Part model, mm, in its own coordinate system. A direction names the side the tool comes from. Round coordinates to 2 decimals unless told otherwise and drop trailing zeros. Loops run counter-clockwise (first coordinate to the right, second up) from the corner with the lowest first, then second, coordinate; pieces in that order, holes last. Notation, with made-up numbers: (11.25, 40) -> (64.25, 40) arc R30 ccw to (64.25, 78) -> close; hole circle Ø1 at (-9, 13). An arc over 180 degrees is marked (long way). Answer as CSV lines item,"result".
from build123d import *

# Parameters (mm, degrees)
BOSS_EXTRUDE1_DEPTH                      = 12.7
SKETCH5_R                                = 3.4544
CUT_EXTRUDE2_DEPTH                       = 31.760138832
SKETCH6_W                                = 19.05
SKETCH6_H                                = 5.55625
SKETCH7_W                                = 19.05
SKETCH7_H                                = 5.55625
CUT_EXTRUDE3_REACH                       = 49.094
SKETCH8_R                                = 2.2479
CUT_EXTRUDE4_DEPTH                       = 48.544988458
MIRROR1_AT_THE_SECOND_PLANE_COPY_1_DEPTH = 48.544988458


with BuildPart() as part:
    # Sketch2 → Boss-Extrude1 (new, symmetric)
    with BuildSketch(Plane(origin=(0, 0, 0), x_dir=(1, 0, 0), z_dir=(0, 1, 0))):
        Polygon((-19.05, 6.35), (19.05, 6.35), (24.972107259, -6.35), (-24.972107259, -6.35), align=None)
    extrude(amount=BOSS_EXTRUDE1_DEPTH, both=True)

    # Sketch5 → Cut-Extrude2 (cut, through all)
    with BuildSketch(Plane.XY.offset(6.35)):
        Circle(SKETCH5_R)
    extrude(amount=-CUT_EXTRUDE2_DEPTH, mode=Mode.SUBTRACT)

    # Sweep1: sweep along a curve in space
    with BuildLine() as sweep1_path:
        Line((-19.05, 12.7, -6.35), (-24.972107259, 12.7, 6.35))
    # Sketch6 → Sweep1 (sweep)
    with BuildSketch(Plane.XY.offset(6.35)):
        with Locations((-34.497107259, 0)):
            Rectangle(SKETCH6_W, SKETCH6_H)
    sweep(path=sweep1_path.line)

    # Sweep2: sweep along a curve in space
    with BuildLine() as sweep2_path:
        Line((24.972107259, 12.7, 6.35), (19.05, 12.7, -6.35))
    # Sketch7 → Sweep2 (sweep)
    with BuildSketch(Plane.XY.offset(6.35)):
        with Locations((34.497107259, 0)):
            Rectangle(SKETCH7_W, SKETCH7_H)
    sweep(path=sweep2_path.line)

    # Sketch8 → Cut-Extrude3 (cut, up to next)
    with BuildSketch(Plane(origin=(0, 2.778125, 0), x_dir=(1, 0, 0), z_dir=(0, 1, 0)), mode=Mode.PRIVATE) as cut_extrude3_sk1:
        with Locations(Location((-32.520728307, 0, 0), (0, 0, 180))):
            Circle(SKETCH8_R)
    cut_extrude3_tool1 = extrude(cut_extrude3_sk1.sketch, amount=-CUT_EXTRUDE3_REACH, mode=Mode.PRIVATE) & part.part
    # Sketch8 → Cut-Extrude3 (cut, up to next)
    with BuildSketch(Plane(origin=(0, 2.778125, 0), x_dir=(1, 0, 0), z_dir=(0, 1, 0)), mode=Mode.PRIVATE) as cut_extrude3_sk2:
        with Locations(Location((32.520728307, 0, 0), (0, 0, 180))):
            Circle(SKETCH8_R)
    cut_extrude3_tool2 = extrude(cut_extrude3_sk2.sketch, amount=-CUT_EXTRUDE3_REACH, mode=Mode.PRIVATE) & part.part
    add(cut_extrude3_tool1.solids().sort_by_distance((-32.520728, 2.778125, 0))[0], mode=Mode.SUBTRACT)
    add(cut_extrude3_tool2.solids().sort_by_distance((32.520728, 2.778125, 0))[0], mode=Mode.SUBTRACT)

    # Sketch9 → Cut-Extrude4 (cut, through all)
    with BuildSketch(Plane.XY.offset(6.35)):
        with BuildLine():
            Line((-24.972107259, 12.7), (-24.972107259, 7.9375))
            Line((-24.972107259, 7.9375), (-18.622107259, 7.9375))
            Line((-18.622107259, 7.9375), (-3.451726858, 12.221930359))
            ThreePointArc((-3.451726858, 12.221930359), (-1.742338148, 12.579914856), (0, 12.7))
            Line((0, 12.7), (-24.972107259, 12.7))
        make_face()
    cut_extrude4 = extrude(amount=-CUT_EXTRUDE4_DEPTH, mode=Mode.SUBTRACT)

    # Mirror1: Cut-Extrude4 across plane
    add(cut_extrude4.mirror(Plane(origin=(0, 0, 0), x_dir=(0, 0, 1), z_dir=(1, 0, 0))), mode=Mode.SUBTRACT)

    # Mirror1 at the second plane: Cut-Extrude4 across plane
    add(cut_extrude4.mirror(Plane.ZX), mode=Mode.SUBTRACT)

    # Mirror1 at the second plane copy 1 sketc → Mirror1 at the second plane copy 1 (cut, through all)
    with BuildSketch(Plane(origin=(0, 0, 6.35), x_dir=(-1, 0, 0), z_dir=(0, 0, 1))):
        with BuildLine():
            Line((-24.972107259, 12.7), (-24.972107259, 7.9375))
            Line((-24.972107259, 7.9375), (-18.622107259, 7.9375))
            Line((-18.622107259, 7.9375), (-3.451726858, 12.221930359))
            ThreePointArc((-3.451726858, 12.221930359), (-1.742338148, 12.579914856), (0, 12.7))
            Line((0, 12.7), (-24.972107259, 12.7))
        make_face()
    extrude(amount=-MIRROR1_AT_THE_SECOND_PLANE_COPY_1_DEPTH, mode=Mode.SUBTRACT)


solid = part.part
Q1. Saw through at B-B, the plane x = 1.5. Write the cut outline in (y, z), then the cut area to 3 significant figures.
Geometry results:
outline,"(-12.61, -6.35) -> (-3.11, -6.35) -> (-3.11, 6.35) -> (-12.61, 6.35) -> close; (3.11, -6.35) -> (12.61, -6.35) -> (12.61, 6.35) -> (3.11, 6.35) -> close"
area,"241 mm2"
Q2. Saw through at D-D, the plane z = -3.25. Write the cut outline in (x, y).
Geometry results:
outline,"(-39.55, -2.78) -> (-20.5, -2.78) -> (-20.5, -7.94) -> (-18.62, -7.94) -> (-3.45, -12.22) arc R12.7 ccw to (3.45, -12.22) -> (18.62, -7.94) -> (20.5, -7.94) -> (20.5, -2.78) -> (39.55, -2.78) -> (39.55, 2.78) -> (20.5, 2.78) -> (20.5, 7.94) -> (18.62, 7.94) -> (3.45, 12.22) arc R12.7 ccw to (-3.45, 12.22) -> (-18.62, 7.94) -> (-20.5, 7.94) -> (-20.5, 2.78) -> (-39.55, 2.78) -> close; hole circle Ø6.91 at (0, 0)"
Q3. Drill centre lines: line 1 along X through (y, z) = (-2.25, 1.25); line 2 along Y through (x, z) = (-19.5, 2.75); line 3 along Y through (x, z) = (-25.5, 0.25). Where is each one in solid material? Low to high.
Geometry results:
line 1,"-41.64 to -34.39, -30.65 to -2.62, 2.62 to 30.65, 34.39 to 41.64"
line 2,"-7.94 to 7.94"
line 3,"-2.78 to 2.78"
Q4. Saw through at A-A, the plane y = 0. Write the cut outline in (x, z), then the cut area to 3 significant figures.
Geometry results:
outline,"(-44.02, 6.35) -> (-38.1, -6.35) -> (-3.45, -6.35) -> (-3.45, 6.35) -> close; (3.45, -6.35) -> (38.1, -6.35) -> (44.02, 6.35) -> (3.45, 6.35) -> close; hole circle Ø4.5 at (-32.52, 0); hole circle Ø4.5 at (32.52, 0)"
area,"923 mm2"
Q5. Drop flat-ended pins along their axis: P1, Ø2, axis at x = -16, z = -2.5, coming from the +Y side; P2, Ø4, axis at x = -34, z = -2.5, coming from the +Y side; P3, Ø4, axis at x = -32.52, z = 0, coming from the -Y side; P4, Ø3, axis at y = -8, z = -0.5, coming from the +X side. Give the stop position or say it passes through.
Geometry results:
P1,"y = 8.96"
P2,"y = 2.78"
P3,"through"
P4,"x = 22.48"
Q6. Which spindle directions (+Z, -Z, +X, -X, +Y, -Y) get a long thin tool onto all of the face, cutting with end or side? Do faces 1 (the face through (-31, 2.778, -3)), 2 (the face through (21, 7.938, 2)), 3 (the face through (29, 2.778, 0)). Say none if no direction does.
Geometry results:
face 1,"-Z, -X, +Y"
face 2,"+Z, -Z, +X, +Y"
face 3,"-Z, +X, +Y"
Q7. Two-plate mould, pull along X, no slides. Class faces 4 (the face through (-11.14, 10.05, 0.09)), 5 (the face through (-0.45, 3.425, 0.089)), 6 (the face through (11.14, 10.05, 0.09)), 7 (the face through (-29, -2.778, 0)): pulls with the +X half, pulls with the -X half, needs draft (parallel to the pull), parting line crosses it, or undercut.
Geometry results:
face 4,"pulls with the -X half"
face 5,"undercut"
face 6,"pulls with the +X half"
face 7,"needs draft"
Q8. Saw through at C-C, the plane z = 0. Give the number of separate pieces and of enclosed holes in the cut face, then the cut area to 3 significant figures.
Geometry results:
separate pieces,"3"
enclosed holes,"1"
area,"1,020 mm2"
